The listing builds one solid part. Answer for the finished solid, in the listing's coordinates (mm). A direction names the side the tool comes from. Round coordinates to 2 decimals unless told otherwise and drop trailing zeros. Loops run counter-clockwise (first coordinate to the right, second up) from the corner with the lowest first, then second, coordinate; pieces in that order, holes last. Notation, with made-up numbers: (46, -21) -> (61, -21) arc R24 ccw to (61, 9) -> close; hole circle Ø3 at (-9.5, 21.5). An arc over 180 degrees is marked (long way). Write each question's results on one line, items separated by ' | '. Start each with the question number.
from build123d import *

# Parameters (mm, degrees)
F1_DEPTH = 631.825
F2_R     = 5.55625
F3_DEPTH = 6.351
F4_R     = 3.96875
F5_DEPTH = 50.801


with BuildPart() as f1:
    # F0 (on Top) → F1 (new body)
    with BuildSketch(Plane.XY):
        Polygon((50.8, 0), (0, 0), (0, -50.8), (6.35, -50.8), (6.35, -6.35), (50.8, -6.35), align=None)
    extrude(amount=F1_DEPTH)

    # F2 (on face) → F3 (cut, through all)
    with BuildSketch(Plane.XZ.offset(6.35)):
        with Locations((25.4, 606.425)):
            Circle(F2_R)
        with Locations((25.4, 25.4)):
            Circle(F2_R)
    extrude(amount=-F3_DEPTH, mode=Mode.SUBTRACT)

    # F4 (on face) → F5 (cut, through all)
    with BuildSketch(Plane(origin=(0, 0, 0), x_dir=(0, -1, 0), z_dir=(-1, 0, 0))):
        with Locations((25.4, 477.8375)):
            Circle(F4_R)
        with Locations((25.4, 153.9875)):
            Circle(F4_R)
        with Locations((25.4, 188.9125)):
            Circle(F4_R)
        with Locations((25.4, 442.9125)):
            Circle(F4_R)
    extrude(amount=-F5_DEPTH, mode=Mode.SUBTRACT)


solid = f1.part
Item 1: The part is cut by section A-A, the plane z = 25.4. Give the vertices of the cut face in (x, y).
Item 2: Each of these flat-tipped pins is pushed along its axis until it touches: pin 1 Ø3 at (y, z) = (-30.5, 131.5) entering from +X; pin 2 Ø1.5 at (x, z) = (41.5, 355.5) entering from -Y. Where does it stop, or does it pass through?
Item 3: Straight lines are drawn through the part: L1, parallel to Z at x = 3, y = -25 (3 decimals); L2, parallel to Z at x = 25.4, y = -1.75 (3 decimals); L3, parallel to Z at x = 1.5, y = -25.4 (3 decimals). For each, find the intervals that lie inside material, in ascending order. Write a range as [from, to].
Item 4: The part is cut by section B-B, the plane x = 25.4. Give the vertices of the cut face in (y, z) (3 decimals), plus the area to 3 significant figures.
Item 5: For faces 1 (the flat face through (28, -6.35, 311)), 2 (the flat face through (26, 0, 311)), determine the directions among +Z, -Z, +X, -X, +Y, -Y from which every point of the face is accessible in a straight line to the end or side of a thin tool.
Item 6: The part is cut by section C-C, the plane y = -41. Give the vertices of the cut face in (x, z) (3 decimals), plus the area to 3 significant figures.
Item 7: Determine the mould class of faces 3 (the flat face through (5, -14, 631.825)), 4 (the cylindrical face through (24.2, -3.2, 601)), 5 (the flat face through (6.35, -29, 311)) for opening direction X: +X half, -X half, draft (parallel to the pull), parting line (faces both ways), or undercut.
Item 8: The part is cut by section D-D, the plane z = 413. Give the vertices of the cut face in (x, y).
Report:
1) outline: (0, -50.8) -> (6.35, -50.8) -> (6.35, -6.35) -> (19.84, -6.35) -> (19.84, 0) -> (0, 0) -> close; (30.96, -6.35) -> (50.8, -6.35) -> (50.8, 0) -> (30.96, 0) -> close
2) pin 1: stops at x = 6.35 | pin 2: stops at y = -6.35
3) L1: z = [0, 150.039], [157.936, 184.964], [192.861, 438.964], [446.861, 473.889], [481.786, 631.825] | L2: z = [0, 19.844], [30.956, 600.869], [611.981, 631.825] | L3: z = [0, 150.019], [157.956, 184.944], [192.881, 438.944], [446.881, 473.869], [481.806, 631.825]
4) outline: (-6.35, 0) -> (0, 0) -> (0, 19.844) -> (-6.35, 19.844) -> close; (-6.35, 30.956) -> (0, 30.956) -> (0, 600.869) -> (-6.35, 600.869) -> close; (-6.35, 611.981) -> (0, 611.981) -> (0, 631.825) -> (-6.35, 631.825) -> close | area: 3,870 mm2
5) face 1: +Z, -Z, +X, -Y | face 2: +Z, -Z, +X, -X, +Y
6) outline: (0, 0) -> (6.35, 0) -> (6.35, 631.825) -> (0, 631.825) -> close | area: 4,010 mm2
7) face 3: draft | face 4: undercut | face 5: +X half
8) outline: (0, -50.8) -> (6.35, -50.8) -> (6.35, -6.35) -> (50.8, -6.35) -> (50.8, 0) -> (0, 0) -> close
